from build123d import *

# Parameters (mm, degrees)
SKETCH2_R                 = 5.65
BOSS_EXTRUDE1_DEPTH       = 1.2
SKETCH3_R                 = 3.825
BOSS_EXTRUDE2_DEPTH       = 2.56
SKETCH5_R                 = 3.9
BOSS_EXTRUDE4_DEPTH       = 0.9
BOSS_EXTRUDE5_DEPTH       = 2.56
FILLET12_R                = 0.3
CIRPATTERN3_COUNT         = 12
FILLET12_OF_CIRPATTERN3_R = 0.3
SKETCH10_R                = 2.3
CUT_EXTRUDE3_DEPTH        = 10.249897297
SKETCH11_R                = 3
CUT_EXTRUDE4_DEPTH        = 0.25


with BuildPart() as part:
    # Sketch2 → Boss-Extrude1 (new body)
    with BuildSketch(Plane(origin=(0, 0, 0), x_dir=(1, 0, 0), z_dir=(0, 1, 0))):
        with Locations(Location((0, 0, 0), (0, 0, 270))):
            Circle(SKETCH2_R)
    extrude(amount=BOSS_EXTRUDE1_DEPTH)

    # Sketch3 → Boss-Extrude2 (add)
    with BuildSketch(Plane(origin=(0, 1.2, 0), x_dir=(1, 0, 0), z_dir=(0, 1, 0))):
        with Locations(Location((0, 0, 0), (0, 0, 90))):
            Circle(SKETCH3_R)
    extrude(amount=BOSS_EXTRUDE2_DEPTH)

    # Sketch5 → Boss-Extrude4 (add)
    with BuildSketch(Plane.XZ):
        with Locations(Location((0, 0, 0), (0, 0, 270))):
            Circle(SKETCH5_R)
    extrude(amount=BOSS_EXTRUDE4_DEPTH)

    # Sketch9 → Boss-Extrude5 (add)
    with BuildSketch(Plane(origin=(0, 1.2, 0), x_dir=(1, 0, 0), z_dir=(0, 1, 0))):
        Polygon((0.39, 2.91), (-0.39, 2.91), (-0.39, 4.74), (0, 4.957049268), (0.39, 4.74), align=None)
    boss_extrude5 = extrude(amount=BOSS_EXTRUDE5_DEPTH)

    # Fillet12
    fillet12_edges = [part.edges().sort_by_distance(p)[0] for p in [
        (-0.39, 2.48, -4.74),
        (0, 2.48, -4.957049268),
        (0.39, 2.48, -4.74),
    ]]
    fillet(fillet12_edges, radius=FILLET12_R)

    # CirPattern3: Boss-Extrude5 ×12 about axis
    cirpattern3_axis = Axis((0, 0, 0), (0, 1, 0))
    for i in range(1, CIRPATTERN3_COUNT):
        add(boss_extrude5.rotate(cirpattern3_axis, i * 360 / CIRPATTERN3_COUNT))

    # Fillet12 of CirPattern3
    fillet12_of_cirpattern3_edges = [part.edges().sort_by_distance(p)[0] for p in [
        (-2.707749907, 2.48, -3.909960414),
        (-2.478524634, 2.48, -4.292930594),
        (-2.032250093, 2.48, -4.299960414),
        (-4.299960414, 2.48, -2.032250093),
        (-4.292930594, 2.48, -2.478524634),
        (-3.909960414, 2.48, -2.707749907),
        (-4.74, 2.48, 0.39),
        (-4.957049268, 2.48, 0),
        (-4.74, 2.48, -0.39),
        (-3.909960414, 2.48, 2.707749907),
        (-4.292930594, 2.48, 2.478524634),
        (-4.299960414, 2.48, 2.032250093),
        (-2.032250093, 2.48, 4.299960414),
        (-2.478524634, 2.48, 4.292930594),
        (-2.707749907, 2.48, 3.909960414),
        (0.39, 2.48, 4.74),
        (0, 2.48, 4.957049268),
        (-0.39, 2.48, 4.74),
        (2.707749907, 2.48, 3.909960414),
        (2.478524634, 2.48, 4.292930594),
        (2.032250093, 2.48, 4.299960414),
        (4.299960414, 2.48, 2.032250093),
        (4.292930594, 2.48, 2.478524634),
        (3.909960414, 2.48, 2.707749907),
        (4.74, 2.48, -0.39),
        (4.957049268, 2.48, 0),
        (4.74, 2.48, 0.39),
        (3.909960414, 2.48, -2.707749907),
        (4.292930594, 2.48, -2.478524634),
        (4.299960414, 2.48, -2.032250093),
        (2.032250093, 2.48, -4.299960414),
        (2.478524634, 2.48, -4.292930594),
        (2.707749907, 2.48, -3.909960414),
    ]]
    fillet(fillet12_of_cirpattern3_edges, radius=FILLET12_OF_CIRPATTERN3_R)

    # Sketch10 → Cut-Extrude3 (cut, through all)
    with BuildSketch(Plane(origin=(0, 3.76, 0), x_dir=(1, 0, 0), z_dir=(0, 1, 0))):
        with Locations(Location((0, 0, 0), (0, 0, 270))):
            Circle(SKETCH10_R)
    extrude(amount=-CUT_EXTRUDE3_DEPTH, mode=Mode.SUBTRACT)

    # Sketch11 → Cut-Extrude4 (cut)
    with BuildSketch(Plane(origin=(0, 3.76, 0), x_dir=(1, 0, 0), z_dir=(0, 1, 0))):
        with Locations(Location((0, 0, 0), (0, 0, 270))):
            Circle(SKETCH11_R)
    extrude(amount=-CUT_EXTRUDE4_DEPTH, mode=Mode.SUBTRACT)


solid = part.part
Build history of the part. All positions in model axes, mm. A direction names the side the tool comes from. Round coordinates to 2 decimals unless told otherwise and drop trailing zeros. Loops run counter-clockwise (first coordinate to the right, second up) from the corner with the lowest first, then second, coordinate; pieces in that order, holes last. Notation, with made-up numbers: (-14, 71) -> (17, 71) arc R5 cw to (17, 76) -> close; hole circle Ø9 at (-27, 17). An arc over 180 degrees is marked (long way). One line per item, written item: value. Start each with the question number.
Q1. Probe line 1 along X through (y, z) = (0.2, 0); line 2 along X through (y, z) = (3.05, 4); line 3 along Y through (x, z) = (3.5, -3.5). List the from-to ranges inside material, lowest first.
Q2. Cut at D-D on y = 1. List the corners of the cut face in (x, z), plus the area to 3 significant figures.
Q3. Cut at C-C on y = -0.25. List the corners of the cut face in (x, z), plus the area to 3 significant figures.
Q4. 3-axis set-ups, long thin cutter, end or side, ignore diameter. For faces 1 (the face through (-1, 2.46, 3.69)), 2 (the face through (1, 2.46, -3.69)), 3 (the face through (-2.7, 2.46, -2.71)), 4 (the face through (3.697, 2.462, -0.982)): which of +Z, -Z, +X, -X, +Y, -Y reach the whole face in a straight line?
Q5. Drop flat-ended pins along their axis: pin 1 Ø1 at (x, z) = (-2.5, -4) entering from -Y; pin 2 Ø2 at (x, y) = (-4, -0.5) entering from -Z; pin 3 Ø5 at (x, z) = (0, 0) entering from +Y; pin 4 Ø4 at (x, z) = (0, 0) entering from +Y. Give the stop position or say it passes through.
Q6. Cut at B-B on z = 0. List the corners of the cut face in (x, y).
Q7. Two-plate mould, pull along Z, no slides. Class faces 5 (the face through (-3.697, 2.462, 0.982)), 6 (the face through (-4, 0, -1)), 7 (the face through (-2.373, -0.444, 3.095)): released by +Z, released by -Z, zero draft, split by the parting line, or undercut.
Q8. Cut at A-A on x = 0. List the corners of the cut face in (y, z).
Computed:
1. line 1: -5.65 to -2.3, 2.3 to 5.65
1. line 2: -2.65 to -1.86, -0.39 to 0.39, 1.86 to 2.65
1. line 3: 0 to 1.2
2. outline: circle Ø11.3 at (0, 0); hole circle Ø4.6 at (0, 0)
2. area: 83.7 mm²
3. outline: circle Ø7.8 at (0, 0); hole circle Ø4.6 at (0, 0)
3. area: 31.2 mm²
4. face 1: +Z, +Y
4. face 2: -Z, +Y
4. face 3: +Y
4. face 4: +X, +Y
5. pin 1: y = 0
5. pin 2: z = -4.7
5. pin 3: y = 3.51
5. pin 4: through
6. outline: (-5.65, 0) -> (-3.9, 0) -> (-3.9, -0.9) -> (-2.3, -0.9) -> (-2.3, 3.51) -> (-3, 3.51) -> (-3, 3.76) -> (-4.91, 3.76) -> (-4.91, 1.2) -> (-5.65, 1.2) -> close; (2.3, -0.9) -> (3.9, -0.9) -> (3.9, 0) -> (5.65, 0) -> (5.65, 1.2) -> (4.91, 1.2) -> (4.91, 3.76) -> (3, 3.76) -> (3, 3.51) -> (2.3, 3.51) -> close
7. face 5: undercut
7. face 6: zero draft
7. face 7: split by the parting line
8. outline: (-0.9, -3.9) -> (0, -3.9) -> (0, -5.65) -> (1.2, -5.65) -> (1.2, -4.91) -> (3.76, -4.91) -> (3.76, -3) -> (3.51, -3) -> (3.51, -2.3) -> (-0.9, -2.3) -> close; (-0.9, 2.3) -> (3.51, 2.3) -> (3.51, 3) -> (3.76, 3) -> (3.76, 4.91) -> (1.2, 4.91) -> (1.2, 5.65) -> (0, 5.65) -> (0, 3.9) -> (-0.9, 3.9) -> close
